Part model, mm, in its own coordinate system. Round coordinates to 2 decimals unless told otherwise and drop trailing zeros. Loops run counter-clockwise (first coordinate to the right, second up) from the corner with the lowest first, then second, coordinate; pieces in that order, holes last. Notation, with made-up numbers: (20.25, -5.75) -> (66.25, -5.75) arc R8 cw to (66.25, -1.75) -> close; hole circle Ø7 at (35, 22.25). An arc over 180 degrees is marked (long way). Use a Markdown table: item, result. Add a question column.
Item 1: Cut at C-C, the plane z = 3.2. List the corners of the cut face in (x, y).
Item 2: Flat gauge pins, fed straight in: pin 1 (2 mm diameter, centred on y = -3.5, z = 0.5, fed in from +X); pin 2 (14 mm diameter, centred on x = -11, y = -11.5, fed in from -Z); pin 3 (1 mm diameter, centred on y = -11, z = 3, fed in from -X). Where does each tip first touch, or does it go through?
Item 3: Cut at A-A, the plane y = 0. List the corners of the cut face in (x, z) (3 decimals), plus the area to 3 significant figures.
Item 4: Probe line 1 (Z direction, x = 16.5, y = -11.5); line 2 (Z direction, x = 21, y = -5.5); line 3 (X direction, y = 11.5, z = 2.2). List the from-to ranges inside material, lowest first. Write a range as [from, to].
Item 5: Cut at B-B, the plane x = 0. List the corners of the cut face in (y, z) (3 decimals), plus the area to 3 significant figures.
```python
from build123d import *

# Parameters (mm, degrees)
PAD_DEPTH    = 1
SKETCH001_R  = 19.92
PAD001_DEPTH = 1
SKETCH002_R  = 23.025
PAD002_DEPTH = 0.65
SKETCH003_R  = 23.025
PAD003_DEPTH = 1.15
FILLET_R     = 1.14


with BuildPart() as part:
    # Sketch → Pad (new body)
    with BuildSketch(Plane.XY):
        with BuildLine():
            ThreePointArc((13.847311, -16.41425), (0, 21.475), (-13.847311, -16.41425))
            ThreePointArc((-6.652084, -23.112353), (-10.16787, -19.675401), (-13.847311, -16.41425))
            Line((-5.5, -24.295), (-6.652084, -23.112353))
            Line((-5.5, -24.295), (5.5, -24.295))
            Line((5.5, -24.295), (6.652084, -23.112353))
            ThreePointArc((13.847311, -16.41425), (10.16787, -19.675401), (6.652084, -23.112353))
        make_face()
    extrude(amount=PAD_DEPTH)

    # Sketch001 (on Face8 of Pad) → Pad001 (join)
    with BuildSketch(Plane.XY.offset(1)):
        Circle(SKETCH001_R)
    extrude(amount=PAD001_DEPTH)

    # Sketch002 (on Face10 of Pad001) → Pad002 (join)
    with BuildSketch(Plane.XY.offset(2)):
        Circle(SKETCH002_R)
    extrude(amount=PAD002_DEPTH)

    # Sketch003 (on Face3 of Pad002) → Pad003 (join)
    with BuildSketch(Plane.XY.offset(2.65)):
        Circle(SKETCH003_R)
    extrude(amount=PAD003_DEPTH)

    # Fillet
    fillet_edges = [part.edges().sort_by_distance(p)[0] for p in [
        (-23.025, 0, 3.8),
    ]]
    fillet(fillet_edges, radius=FILLET_R)


solid = part.part
```
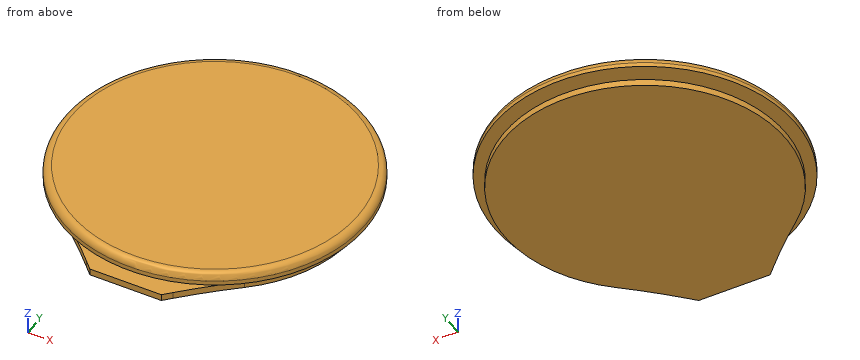
A:
| question | item | result |
|---|---|---|
| 1 | outline | circle Ø45.78 at (0, 0) |
| 2 | pin 1 | stops at x = 21.33 |
| 2 | pin 2 | stops at z = 0 |
| 2 | pin 3 | stops at x = -20.46 |
| 3 | outline | (-23.025, 2) -> (-19.92, 2) -> (-19.92, 1) -> (-21.475, 1) -> (-21.475, 0) -> (21.475, 0) -> (21.475, 1) -> (19.92, 1) -> (19.92, 2) -> (23.025, 2) -> (23.025, 2.66) arc R1.14 ccw to (21.885, 3.8) -> (-21.885, 3.8) arc R1.14 ccw to (-23.025, 2.66) -> close |
| 3 | area | 165 mm^2 |
| 4 | line 1 | z = [0, 1], [2, 3.8] |
| 4 | line 2 | z = [2, 3.8] |
| 4 | line 3 | x = [-19.95, 19.95] |
| 5 | outline | (-24.295, 0) -> (21.475, 0) -> (21.475, 1) -> (19.92, 1) -> (19.92, 2) -> (23.025, 2) -> (23.025, 2.66) arc R1.14 ccw to (21.885, 3.8) -> (-21.885, 3.8) arc R1.14 ccw to (-23.025, 2.66) -> (-23.025, 2) -> (-19.92, 2) -> (-19.92, 1) -> (-24.295, 1) -> close |
| 5 | area | 168 mm^2 |
